Geometry: final body of the model. Coordinates: model frame, mm. Face numbers are marked on the shaded views. A direction names the side the tool comes from. Round coordinates to 2 decimals unless told otherwise and drop trailing zeros. Loops run counter-clockwise (first coordinate to the right, second up) from the corner with the lowest first, then second, coordinate; pieces in that order, holes last. Notation, with made-up numbers: M 34,28 L 73,28 A34 cw 73,62 Z; hole C 11.25,39 d8. An arc over 180 degrees is marked long. Answer as a JSON object with one key per item and string values.
from build123d import *

# Parameters (mm, degrees)
BOSS_EXTRUDE1_DEPTH = 1.5
SKETCH3_W           = 2
SKETCH3_H           = 17
BOSS_EXTRUDE2_DEPTH = 20
CUT_EXTRUDE1_DEPTH  = 5.680224753
CUT_EXTRUDE2_DEPTH  = 5.680224753


with BuildPart() as part:
    # Sketch1 → Boss-Extrude1 (new body)
    with BuildSketch(Plane.XY):
        with BuildLine():
            Line((-1, 8.5), (1, 8.5))
            ThreePointArc((1, 8.5), (3.121320344, 7.621320344), (4, 5.5))
            Line((4, 5.5), (4, -5.5))
            ThreePointArc((4, -5.5), (3.121320344, -7.621320344), (1, -8.5))
            Line((1, -8.5), (-1, -8.5))
            ThreePointArc((-1, -8.5), (-3.121320344, -7.621320344), (-4, -5.5))
            Line((-4, -5.5), (-4, 5.5))
            ThreePointArc((-4, 5.5), (-3.121320344, 7.621320344), (-1, 8.5))
        make_face()
    extrude(amount=BOSS_EXTRUDE1_DEPTH)

    # Sketch3 → Boss-Extrude2 (add)
    with BuildSketch(Plane(origin=(0, 0, 0), x_dir=(-1, 0, 0), z_dir=(0, 0, -1))):
        with Locations((0.319775247, 0)):
            Rectangle(SKETCH3_W, SKETCH3_H)
    extrude(amount=BOSS_EXTRUDE2_DEPTH)

    # Sketch4 → Cut-Extrude1 (cut, through all)
    with BuildSketch(Plane(origin=(0.680224753, 0, 0), x_dir=(0, 0, -1), z_dir=(1, 0, 0))):
        Polygon((0, -8.5), (10.392304845, -2.5), (0, 8.5), (20, 8.5), (20, -8.5), align=None)
    extrude(amount=-CUT_EXTRUDE1_DEPTH, mode=Mode.SUBTRACT)

    # Sketch5 → Cut-Extrude2 (cut, through all)
    with BuildSketch(Plane(origin=(0.680224753, 0, 0), x_dir=(0, 0, -1), z_dir=(1, 0, 0))):
        Polygon((2, 3.470750697), (2, -5.035898385), (7.200217087, -2.03355165), align=None)
    extrude(amount=-CUT_EXTRUDE2_DEPTH, mode=Mode.SUBTRACT)


solid = part.part
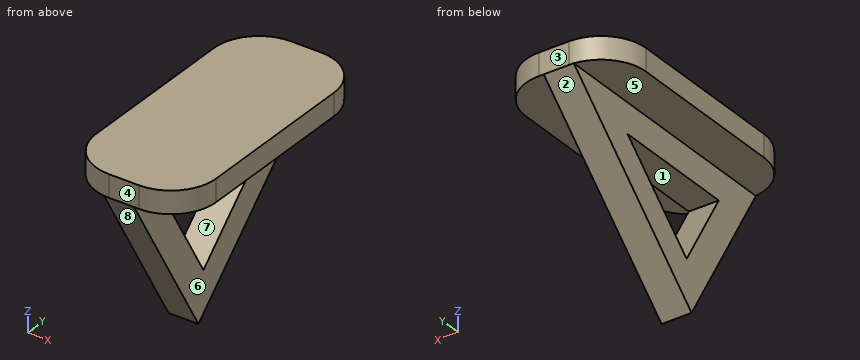
1) Ray query, line 1 (Z direction, x = 3, y = 3.75); line 2 (X direction, y = -3.25, z = -1); line 3 (Y direction, x = -0.25, z = -4.25). Return the intervals inside material, ascending.
Results:
{"line 1": "0 to 1.5", "line 2": "-1.32 to 0.68", "line 3": "-6.05 to -3.74, 1.09 to 4"}
2) Section query B-B (x = 0). Return the cut outline in (y, z).
Results:
{"outline": "M -8.5,0 L -2.5,-10.39 L 8.5,0 L 8.5,1.5 L -8.5,1.5 Z; hole M -5.04,-2 L -2.03,-7.2 L 3.47,-2 Z"}
3) Section query C-C (z = -5). Return the cut outline in (x, y).
Results:
{"outline": "M -1.32,-5.61 L 0.68,-5.61 L 0.68,-3.3 L -1.32,-3.3 Z; M -1.32,0.3 L 0.68,0.3 L 0.68,3.21 L -1.32,3.21 Z"}
4) Pull-direction query (Z, two-part tool) for the marked faces 1, 2 and 3; classes: +Z half, -Z half, draft (parallel to the pull), parting line (faces both ways), or undercut.
Results:
{"face 1": "undercut", "face 2": "-Z half", "face 3": "draft"}
5) Reachability of the marked faces 4, 5, 6, 7 and 8 from +Z, -Z, +X, -X, +Y, -Y: full face, straight path, thin tool, end or side. Return the list, or none.
Results:
{"face 4": "+Z, -Z, +X, -X, -Y", "face 5": "-Z, -X, +Y, -Y", "face 6": "-Z, +X, +Y, -Y", "face 7": "+X, -X", "face 8": "-Z, +X, -X, -Y"}
6) Section query D-D (y = -7.25). Return the cut outline in (x, z).
Results:
{"outline": "M -3.44,0 L -1.32,0 L -1.32,-2.17 L 0.68,-2.17 L 0.68,0 L 3.44,0 L 3.44,1.5 L -3.44,1.5 Z"}
7) Section query A-A (y = -0.75). Return the cut outline in (x, z), and give its area (3 significant figures).
Results:
{"outline": "M -4,0 L -1.32,0 L -1.32,-2 L 0.68,-2 L 0.68,0 L 4,0 L 4,1.5 L -4,1.5 Z; M -1.32,-8.74 L 0.68,-8.74 L 0.68,-5.99 L -1.32,-5.99 Z", "area": "21.5 mm2"}
8) Pin query (flat end, axial travel): P1, Ø2, axis at y = 2.5, z = -6, coming from the +X side; P2, Ø4, axis at x = 0.5, z = -7.5, coming from the -Y side; P3, Ø3, axis at y = 5.5, z = -2.5, coming from the -X side. Return the tip coordinate at first contact, or that it passes through.
Results:
{"P1": "x = 0.68", "P2": "y = -5.32", "P3": "x = -1.32"}
